Build history of the part. All positions in model axes, mm. A direction names the side the tool comes from. Give positions to 0.01 mm unless a question says otherwise; leave off trailing zeros. Loops run counter-clockwise (first coordinate to the right, second up) from the corner with the lowest first, then second, coordinate; pieces in that order, holes last. Notation, with made-up numbers: M 32,-7 L 66,-7 A17 ccw 66,15 Z; hole C 9.5,-3 d2. An arc over 180 degrees is marked long. Answer as a JSON object with one key per item and string values. Group by question number.
1. Slice it at A-A (y = -9.5). List the corners of the cut face in (x, z), then the cut area to 3 significant figures.
2. Drop flat-ended pins along their axis: pin 1 Ø13.5 at (y, z) = (14.5, -7.5) entering from +X; pin 2 Ø24.5 at (x, y) = (16.66, -13.35) entering from +Z; pin 3 Ø13.5 at (x, y) = (-16.87, -12.95) entering from -Z; pin 4 Ø2 at (y, z) = (14, 7) entering from +X. Give the stop position or say it passes through.
3. 3-axis set-ups, long thin cutter, end or side, ignore diameter. For faces 1 (the face through (-2, -13, -16.765)), 2 (the face through (-46.56, -17.79, -8.5)), 3 (the face through (66.548, 11, 17)), 4 (the face through (66.859, -13, -8)), 5 (the face through (-68.064, -13, -8)): which of +Z, -Z, +X, -X, +Y, -Y reach the whole face in a straight line?
4. Slice it at D-D (y = -16). List the corners of the cut face in (x, z), then the cut area to 3 significant figures.
5. Mould opens along X. For faces 6 (the face through (42.955, -16.069, -8.5)), 7 (the face through (-68.072, 11, 17)), 8 (the face through (0, 21.719, 16)) say: released by +X, released by -X, zero draft, split by the parting line, or undercut.
6. Drill centre lines: line 1 along X through (y, z) = (5, 2.5); line 2 along X through (y, z) = (8, -0.5); line 3 along Z through (x, y) = (25.5, -13). Where is each one in solid material? Low to high. Write a range as [from, to].
7. Slice it at C-C (z = -12.5). List the corners of the cut face in (x, y).
8. Slice it at B-B (x = 11). List the corners of the cut face in (y, z), then the cut area to 3 significant figures.
from build123d import *

# Parameters (mm, degrees)
F0_W     = 134.9227651954
F0_H     = 16.7649574578
F1_DEPTH = 25.4
F2_W     = 21.8847934157
F2_H     = 16.9657338411
F3_DEPTH = 25.4
F4_DEPTH = 25.4
F5_DEPTH = 16.002
F6_DEPTH = 68.326
F7_W     = 21.7192191631
F7_H     = 33.0388583243
F8_DEPTH = 66.548
F9_DEPTH = 68.072
F11_D    = 15.24
F12_D    = 15.24
F13_D    = 15.24


with BuildPart() as f1:
    # F0 (on Front) → F1 (new body)
    with BuildSketch(Plane.XZ):
        with Locations((-0.6023310125, -8.3824787289)):
            Rectangle(F0_W, F0_H)
    extrude(amount=F1_DEPTH)

    # F2 (on Right) → F3 (join)
    with BuildSketch(Plane.YZ):
        with Locations((10.9423967078, -8.4828669205)):
            Rectangle(F2_W, F2_H)
    extrude(amount=F3_DEPTH)

    # F4 (add): a face of the model
    f4_faces = [f1.faces().sort_by_distance(p)[0] for p in [
        (25.4, 10.9423967078, -8.4828669205),
    ]]
    extrude(f4_faces, amount=F4_DEPTH)

    # F5 (add): a face of the model
    f5_faces = [f1.faces().sort_by_distance(p)[0] for p in [
        (50.8, 10.9423967078, -8.4828669205),
    ]]
    extrude(f5_faces, amount=F5_DEPTH)

    # F6 (add): a face of the model
    f6_faces = [f1.faces().sort_by_distance(p)[0] for p in [
        (0, 10.9423967078, -8.4828669205),
    ]]
    extrude(f6_faces, amount=F6_DEPTH)

    # F7 (on Right) → F8 (join)
    with BuildSketch(Plane.YZ):
        with Locations((10.8596095815, 16.5194291621)):
            Rectangle(F7_W, F7_H)
    extrude(amount=F8_DEPTH)

    # F9 (add): a face of the model
    f9_faces = [f1.faces().sort_by_distance(p)[0] for p in [
        (0, 10.8596095815, 16.5194291621),
    ]]
    extrude(f9_faces, amount=F9_DEPTH)

    # F11 (through all)
    with Locations(Plane.XY):
        with Locations((-52.6038147509, -13.1509546191)):
            Hole(F11_D / 2)

    # F12 (through all)
    with Locations(Plane.XY):
        with Locations((-16.8653447181, -12.9501754418)):
            Hole(F12_D / 2)

    # F13 (through all)
    with Locations(Plane.XY):
        with Locations((16.6645683348, -13.3517310023), (49.9937050045, -13.1509546191)):
            Hole(F13_D / 2)


solid = f1.part
Established:
{
 "1": {"outline": "M -68.06,-16.76 L -59.29,-16.76 L -59.29,0 L -68.06,0 Z; M -45.92,-16.76 L -23.66,-16.76 L -23.66,0 L -45.92,0 Z; M -10.07,-16.76 L 10.09,-16.76 L 10.09,0 L -10.07,0 Z; M 23.24,-16.76 L 43.31,-16.76 L 43.31,0 L 23.24,0 Z; M 56.68,-16.76 L 66.86,-16.76 L 66.86,0 L 56.68,0 Z", "area": "1,370 mm^2"},
 "2": {"pin 1": "stops at x = 66.8", "pin 2": "stops at z = 0", "pin 3": "passes through", "pin 4": "stops at x = 66.55"},
 "3": {"face 1": "-Z, +X, -X, -Y", "face 2": "+Z, -Z", "face 3": "+Z, +X, +Y, -Y", "face 4": "+Z, -Z, +X, +Y, -Y", "face 5": "+Z, -Z, -X, -Y"},
 "4": {"outline": "M -68.06,-16.76 L -59.67,-16.76 L -59.67,0 L -68.06,0 Z; M -45.54,-16.76 L -23.85,-16.76 L -23.85,0 L -45.54,0 Z; M -9.88,-16.76 L 9.52,-16.76 L 9.52,0 L -9.88,0 Z; M 23.81,-16.76 L 42.93,-16.76 L 42.93,0 L 23.81,0 Z; M 57.06,-16.76 L 66.86,-16.76 L 66.86,0 L 57.06,0 Z", "area": "1,310 mm^2"},
 "5": {"face 6": "undercut", "face 7": "released by -X", "face 8": "zero draft"},
 "6": {"line 1": "x = [-68.07, 66.55]", "line 2": "x = [-68.33, 66.8]", "line 3": "z = [-16.76, 0]"},
 "7": {"outline": "M -68.33,0 L -68.06,0 L -68.06,-25.4 L 66.86,-25.4 L 66.86,0 L 66.8,0 L 66.8,21.88 L -68.33,21.88 Z; hole C -52.6,-13.15 d15.24; hole C -16.87,-12.95 d15.24; hole C 16.66,-13.35 d15.24; hole C 49.99,-13.15 d15.24"},
 "8": {"outline": "M -25.4,-16.76 L -18.45,-16.76 L -18.45,0 L -25.4,0 Z; M -8.25,-16.76 L 0,-16.76 L 0,-16.97 L 21.88,-16.97 L 21.88,0 L 21.72,0 L 21.72,33.04 L 0,33.04 L 0,0 L -8.25,0 Z", "area": "1,340 mm^2"}
}
